```python
from build123d import *

# Parameters (mm, degrees)
SKETCH_1_W             = 113
SKETCH_1_H             = 50
EXTRUDE_1_DEPTH        = 5
SKETCH_2_R             = 1.575
CUT_EXTRUDE_610_DEPTH  = 4.2
SKETCH_3_R             = 1.575
CUT_EXTRUDE_919_DEPTH  = 4.2
SKETCH_4_W             = 5
SKETCH_4_H             = 46
CUT_EXTRUDE_1430_DEPTH = 1.2
SKETCH_5_R             = 3.35
SMA_DEPTH              = 116.840407458
SKETCH_6_R             = 5
SMA_2_DEPTH            = 2
SKETCH_7_W             = 12
SKETCH_7_H             = 36.84
SMA_3_DEPTH            = 2
CHAMFER_2760_SIZE      = 0.5


with BuildPart() as part:
    # Эскиз1 → Бобышка-Вытянуть1 (new body)
    with BuildSketch(Plane(origin=(0, 0, 0), x_dir=(0, 0, -1), z_dir=(1, 0, 0))):
        with Locations((-56.5, 0)):
            Rectangle(SKETCH_1_W, SKETCH_1_H)
    extrude(amount=EXTRUDE_1_DEPTH)

    # Эскиз2 → Cut-Extrude 610 (cut)
    with BuildSketch(Plane.XZ.offset(25)):
        with Locations(Location((2.5, 94.166666667, 0), (0, 0, 270))):
            Circle(SKETCH_2_R)
        with Locations(Location((2.5, 75.333333333, 0), (0, 0, 270))):
            Circle(SKETCH_2_R)
        with Locations(Location((2.5, 56.5, 0), (0, 0, 270))):
            Circle(SKETCH_2_R)
        with Locations(Location((2.5, 37.666666667, 0), (0, 0, 270))):
            Circle(SKETCH_2_R)
        with Locations(Location((2.5, 18.833333333, 0), (0, 0, 270))):
            Circle(SKETCH_2_R)
    cut_extrude_610 = extrude(amount=-CUT_EXTRUDE_610_DEPTH, mode=Mode.SUBTRACT)

    # Зеркальное отражение1: Cut-Extrude 610 across plane
    add(cut_extrude_610.mirror(Plane(origin=(0, 0, 0), x_dir=(0, 0, 1), z_dir=(0, -1, 0))), mode=Mode.SUBTRACT)

    # Эскиз3 → Cut-Extrude 919 (cut)
    with BuildSketch(Plane.XY.offset(113)):
        with Locations((2.5, 15)):
            Circle(SKETCH_3_R)
        with Locations((2.5, 0)):
            Circle(SKETCH_3_R)
        with Locations((2.5, -15)):
            Circle(SKETCH_3_R)
    cut_extrude_919 = extrude(amount=-CUT_EXTRUDE_919_DEPTH, mode=Mode.SUBTRACT)

    # Зеркальное отражение2: Cut-Extrude 919 across plane
    add(cut_extrude_919.mirror(Plane(origin=(0, 0, 56.5), x_dir=(1, 0, 0), z_dir=(0, 0, -1))), mode=Mode.SUBTRACT)

    # Эскиз4 → Cut-Extrude 1430 (cut)
    with BuildSketch(Plane(origin=(5, 0, 0), x_dir=(0, 0, -1), z_dir=(1, 0, 0))):
        with Locations((-10.4, 0)):
            Rectangle(SKETCH_4_W, SKETCH_4_H)
        with Locations((-33.4, 0)):
            Rectangle(SKETCH_4_W, SKETCH_4_H)
        with Locations((-58.4, 0)):
            Rectangle(SKETCH_4_W, SKETCH_4_H)
        with Locations((-72.03, 0)):
            Rectangle(SKETCH_4_W, SKETCH_4_H)
        with Locations((-97.35, 0)):
            Rectangle(SKETCH_4_W, SKETCH_4_H)
    extrude(amount=-CUT_EXTRUDE_1430_DEPTH, mode=Mode.SUBTRACT)

    # Эскиз5 → SMA раземы (cut, through all)
    with BuildSketch(Plane(origin=(5, 0, 0), x_dir=(0, 0, -1), z_dir=(1, 0, 0))):
        with Locations((-86.68, 11.54)):
            Circle(SKETCH_5_R)
        with Locations((-86.68, -0.09)):
            Circle(SKETCH_5_R)
        with Locations((-86.68, -13.3)):
            Circle(SKETCH_5_R)
    extrude(amount=-SMA_DEPTH, mode=Mode.SUBTRACT)

    # Эскиз6 → SMA раземы2 (cut)
    with BuildSketch(Plane.ZY):
        with Locations((86.68, 11.54)):
            Circle(SKETCH_6_R)
        with Locations((86.68, -0.09)):
            Circle(SKETCH_6_R)
        with Locations((86.68, -13.3)):
            Circle(SKETCH_6_R)
    extrude(amount=-SMA_2_DEPTH, mode=Mode.SUBTRACT)

    # Эскиз7 → SMA раземы3 (cut)
    with BuildSketch(Plane(origin=(5, 0, 0), x_dir=(0, 0, -1), z_dir=(1, 0, 0))):
        with Locations((-86.68, -0.88)):
            Rectangle(SKETCH_7_W, SKETCH_7_H)
    extrude(amount=-SMA_3_DEPTH, mode=Mode.SUBTRACT)

    # Chamfer 2760
    chamfer_2760_edges = [part.edges().sort_by_distance(p)[0] for p in [
        (2.5, -25, 95.741666667),
        (2.5, -25, 76.908333333),
        (2.5, -25, 58.075),
        (2.5, -25, 39.241666667),
        (2.5, -25, 20.408333333),
        (2.5, 25, 95.741666667),
        (2.5, 25, 76.908333333),
        (2.5, 25, 58.075),
        (2.5, 25, 39.241666667),
        (2.5, 25, 20.408333333),
        (0.925, 15, 113),
        (0.925, 0, 113),
        (0.925, -15, 113),
        (0.925, 15, 0),
        (0.925, 0, 0),
        (0.925, -15, 0),
    ]]
    chamfer(chamfer_2760_edges, length=CHAMFER_2760_SIZE)


solid = part.part
```
Check sheet for the modelled part. Datum: model origin and axes. Units: mm. A direction names the side the tool comes from. Give positions to 0.01 mm unless a question says otherwise; leave off trailing zeros. Order: outer loops, then holes, each group sorted by start corner. A loop starts at its lowest first (then second) coordinate and runs counter-clockwise, first axis right, second up. Notation, with made-up numbers: (-6.75, -23) -> (-0.75, -23) arc R17 ccw to (-0.75, 10) -> close; hole circle Ø11 at (43.5, 40). An arc over 180 degrees is marked (long way). Use CSV: the item, a comma, the result in double quotes. Start each with the question number.
1) Sectioned sample at B-B, the plane z = 86.68. Give the number of separate pieces and of enclosed holes in the cut face, plus the area to 3 significant figures.
2) Sectioned sample at A-A, the plane z = 34. Record the boundary of the cut face in (x, y).
3) Go/stop test with flat-tipped pins: P1, Ø2.5, axis at y = -1.5, z = 96.5, coming from the +X side; P2, Ø2.5, axis at x = 2.5, y = 15, coming from the +Z side; P3, Ø0.9, axis at x = 2, z = 38.5, coming from the +Y side. Record where each tip stops, or that it passes through.
4) Mould release check, pull along X, two halves, no side actions. Record for faces 1 (the face through (2.973, 22.676, 36.164)), 2 (the face through (2, -3.4, 85.5)), 3 (the face through (0.986, 9.625, 91.299)), 4 (the face through (3, 20.8, 19)): released by +X, released by -X, zero draft, split by the parting line, or undercut.
5) Material ranges on line 1 (Y direction, x = 2.5, z = 3.2) (3 decimals); line 2 (Z direction, x = 2.55, y = 21); line 3 (Y direction, x = 2.6, z = 86.68), recorded low to high. Write a range as from..to.
6) Set-up check for faces 5 (the face through (2, -15, 108.8)), 6 (the face through (0.96, 22.68, 75.67)), 7 (the face through (3.8, 0, 10)), 8 (the face through (3, -20.8, 38)), 9 (the face through (0.2, -25, 57.3)): record each of +Z, -Z, +X, -X, +Y, -Y from which the full face is reachable in a straight line by a thin tool's end or side.
Recorded:
1,separate pieces,"4"
1,enclosed holes,"0"
1,area,"96.2 mm2"
2,outline,"(0, -25) -> (5, -25) -> (5, -23) -> (3.8, -23) -> (3.8, 23) -> (5, 23) -> (5, 25) -> (0, 25) -> close"
3,P1,"x = 3.8"
3,P2,"z = 108.8"
3,P3,"y = 20.8"
4,face 1,"undercut"
4,face 2,"released by -X"
4,face 3,"zero draft"
4,face 4,"undercut"
5,line 1,"-25..-16.575, -13.425..-1.575, 1.575..13.425, 16.575..25"
5,line 2,"0..17.26, 20.41..36.09, 39.24..54.93, 58.07..73.76, 76.91..92.59, 95.74..113"
5,line 3,"-25..-16.65, -9.95..-3.44, 3.26..8.19, 14.89..25"
6,face 5,"+Z"
6,face 6,"+Y"
6,face 7,"+X"
6,face 8,"-Y"
6,face 9,"+Z, -Z, +X, -X, -Y"
